from build123d import *

# Parameters (mm, degrees)
SKETCH1_W           = 90
SKETCH1_H           = 80
BOSS_EXTRUDE4_DEPTH = 70
BOSS_EXTRUDE5_DEPTH = 90
SKETCH9_R           = 2.5
SKETCH9_R_2         = 1.4
BOSS_EXTRUDE6_DEPTH = 90
SKETCH10_W          = 66
SKETCH10_H          = 76
CUT_EXTRUDE1_DEPTH  = 134.541756472
CUT_EXTRUDE2_DEPTH  = 134.541756472
SKETCH16_W          = 90
SKETCH16_H          = 30
CUT_EXTRUDE3_DEPTH  = 10


with BuildPart() as part:
    # Sketch1 → Boss-Extrude4 (new body)
    with BuildSketch(Plane.XY):
        Rectangle(SKETCH1_W, SKETCH1_H)
    extrude(amount=BOSS_EXTRUDE4_DEPTH)

    # Sketch8 → Boss-Extrude5 (add, through all)
    with BuildSketch(Plane.ZY.offset(45)):
        Polygon((70, 40), (85.852498999, 0), (70, -40), align=None)
    extrude(amount=-BOSS_EXTRUDE5_DEPTH)

    # Sketch9 → Boss-Extrude6 (add, through all)
    with BuildSketch(Plane.ZY.offset(45)):
        with Locations((87.685368667, 0)):
            Circle(SKETCH9_R)
        with Locations(Location((87.685368667, 0, 0), (0, 0, 270))):
            Circle(SKETCH9_R_2, mode=Mode.SUBTRACT)
    extrude(amount=-BOSS_EXTRUDE6_DEPTH)

    # Sketch10 → Cut-Extrude1 (cut, through all)
    with BuildSketch(Plane.ZY.offset(45)):
        with Locations((35, 0)):
            Rectangle(SKETCH10_W, SKETCH10_H)
    extrude(amount=-CUT_EXTRUDE1_DEPTH, mode=Mode.SUBTRACT)

    # Sketch11 → Cut-Extrude2 (cut, through all)
    with BuildSketch(Plane(origin=(45, 0, 0), x_dir=(0, 0, -1), z_dir=(1, 0, 0))):
        Polygon((-68.641168629, 38.000299069), (-83.701161204, 0), (-68.640413999, -38.002203199), (-68, -38), (-68, 38), align=None)
    extrude(amount=-CUT_EXTRUDE2_DEPTH, mode=Mode.SUBTRACT)

    # Sketch16 → Cut-Extrude3 (cut)
    with BuildSketch(Plane(origin=(0, 0, 0), x_dir=(-1, 0, 0), z_dir=(0, 0, -1))):
        Rectangle(SKETCH16_W, SKETCH16_H)
    extrude(amount=-CUT_EXTRUDE3_DEPTH, mode=Mode.SUBTRACT)


solid = part.part
Geometry: final body of the model. Coordinates: model frame, mm. A direction names the side the tool comes from. Give positions to 0.01 mm unless a question says otherwise; leave off trailing zeros. Order: outer loops, then holes, each group sorted by start corner. A loop starts at its lowest first (then second) coordinate and runs counter-clockwise, first axis right, second up. Notation, with made-up numbers: (34.25, -20.5) -> (69.25, -20.5) arc R24 cw to (69.25, -3.5) -> close; hole circle Ø7 at (85, 80.25). An arc over 180 degrees is marked (long way). Put each result on its own line as item: value.
Q1. Draft query along Y for faces 3 (the face through (-1, -40, 35)), 4 (the face through (-1, -27, 2)), 5 (the face through (45, 39, 38)). Return one class per face: released by +Y, released by -Y, zero draft, split by the parting line, or undercut.
Here are the results:
face 3: released by -Y
face 4: undercut
face 5: zero draft
Q2. Section B-B, the plane y = -19.5. Return loops of the section in (x, z).
Here are the results:
outline: (-45, 0) -> (45, 0) -> (45, 2) -> (-45, 2) -> close; (-45, 75.97) -> (45, 75.97) -> (45, 78.12) -> (-45, 78.12) -> close
Q3. Material intervals for L1, parallel to Y at x = 0, z = 62; L2, parallel to Z at x = 13, y = 0; L3, parallel to Z at x = 4, y = 28.5, sorted ascending.
Here are the results:
L1: y = -40 to -38, 38 to 40
L2: z = 83.7 to 86.29, 89.09 to 90.19
L3: z = 0 to 2, 72.41 to 74.56
Q4. Section A-A, the plane z = 64. Return loops of the section in (x, y), then the cut area to 3 significant figures.
Here are the results:
outline: (-45, -40) -> (45, -40) -> (45, -38) -> (-45, -38) -> close; (-45, 38) -> (45, 38) -> (45, 40) -> (-45, 40) -> close
area: 360 mm^2
Q5. Section D-D, the plane y = -6.5. Return loops of the section in (x, z), then the cut area to 3 significant figures.
Here are the results:
outline: (-45, 81.13) -> (45, 81.13) -> (45, 83.28) -> (-45, 83.28) -> close
area: 194 mm^2
Q6. Pin query (flat end, axial travel): pin 1 (12 mm diameter, centred on x = -35.5, y = 28, fed in from +Z); pin 2 (6 mm diameter, centred on x = -31.5, y = 13, fed in from +Z); pin 3 (10 mm diameter, centred on x = -1.5, y = -5.5, fed in from +Z). Return the tip coordinate at first contact, or that it passes through.
Here are the results:
pin 1: stops at z = 77.13
pin 2: stops at z = 81.89
pin 3: stops at z = 90.13
Q7. Reachability of faces 1 (the face through (-1, -38, 35)), 2 (the face through (-1, 40, 35)) from +Z, -Z, +X, -X, +Y, -Y: full face, straight path, thin tool, end or side. Return the list, or none.
Here are the results:
face 1: +X, -X
face 2: +Z, -Z, +X, -X, +Y
Q8. Section C-C, the plane x = 15.5. Return loops of the section in (y, z).
Here are the results:
outline: (-40, 0) -> (-15, 0) -> (-15, 2) -> (-38, 2) -> (-38, 68) -> (-38, 68.64) -> (0, 83.7) -> (38, 68.64) -> (38, 68) -> (38, 2) -> (15, 2) -> (15, 0) -> (40, 0) -> (40, 70) -> (1.07, 85.43) arc R2.5 ccw (long way) to (-1.07, 85.43) -> (-40, 70) -> close; hole circle Ø2.8 at (0, 87.69)
